Geometry: final body of the model. Coordinates: model frame, mm. A direction names the side the tool comes from. Coordinates: 2 decimals unless noted, no trailing zeros. Order: outer loops, then holes, each group sorted by start corner. A loop starts at its lowest first (then second) coordinate and runs counter-clockwise, first axis right, second up. Notation, with made-up numbers: M 71,23.5 L 85,23.5 A30 ccw 85,56.5 Z; hole C -2.75,-10.5 d7. An arc over 180 degrees is marked long. One line per question, with ' | ' between items.
from build123d import *

# Parameters (mm, degrees)
SKETCH1_R           = 3.7338
SKETCH1_R_2         = 2.6797
BOSS_EXTRUDE1_DEPTH = 1.1176
SHELL1_T            = -0.5715
BOSS_EXTRUDE2_DEPTH = 0.5588
SKETCH4_R           = 2.615046293
SKETCH4_R_2         = 2.107046293
BOSS_EXTRUDE3_DEPTH = 1.1176
BOSS_EXTRUDE4_DEPTH = 0.508
SKETCH7_W           = 0.381
SKETCH7_H           = 0.933727322


with BuildPart() as part:
    # Sketch1 → Boss-Extrude1 (new body)
    with BuildSketch(Plane(origin=(0, 0, 0), x_dir=(1, 0, 0), z_dir=(0, 1, 0))):
        with Locations(Location((0, 0, 0), (0, 0, 270))):
            Circle(SKETCH1_R)
        with Locations(Location((0, 0, 0), (0, 0, 270))):
            Circle(SKETCH1_R_2, mode=Mode.SUBTRACT)
    extrude(amount=-BOSS_EXTRUDE1_DEPTH)


with BuildPart() as body_2:
    # Sketch2 → Revolve1 (revolve)
    with BuildSketch(Plane.XY):
        with BuildLine():
            Line((0, -1.1176), (0, -20.9296))
            ThreePointArc((0, -20.9296), (-0.789505828, -20.640890822), (-1.206518449, -19.910977871))
            Line((-1.206518449, -19.910977871), (-2.770770199, -10.714786652))
            ThreePointArc((-2.770770199, -10.714786652), (-2.859495986, -10.068144543), (-2.906518408, -9.4171398))
            Line((-2.906518408, -9.4171398), (-3.2385, -1.1176))
            Line((-3.2385, -1.1176), (0, -1.1176))
        make_face()
    revolve(axis=Axis((0, -1.1176, 0), (0, -1, 0)))

    # Shell1
    shell1_openings = [body_2.faces().sort_by_distance(p)[0] for p in [
        (0, -1.1176, 0),
    ]]
    offset(amount=SHELL1_T, openings=shell1_openings, kind=Kind.INTERSECTION)


with BuildPart() as part_1:
    add(part.part)

    # Combine1: union body 2
    add(body_2.part)

    # Sketch3 → Boss-Extrude2 (add, symmetric)
    with BuildSketch(Plane.XY):
        with BuildLine():
            Line((3.7338, -1.1176), (4.365322861, -1.1176))
            Line((4.365322861, -1.1176), (5.180035681, -1.1176))
            ThreePointArc((5.180035681, -1.1176), (6.050241958, -0.247393722), (5.180035681, 0.622812555))
            Line((5.180035681, 0.622812555), (4.365322861, 0.622812555))
            Line((4.365322861, 0.622812555), (3.379294532, 0.622812555))
            Line((3.379294532, 0.622812555), (3.379294532, 0.112660745))
            Line((3.379294532, 0.112660745), (4.365322861, 0.112660745))
            Line((4.365322861, 0.112660745), (4.365322861, 0.36773665))
            Line((4.365322861, 0.36773665), (5.180035681, 0.36773665))
            ThreePointArc((5.180035681, 0.36773665), (5.795166053, -0.247393722), (5.180035681, -0.862524095))
            Line((5.180035681, -0.862524095), (4.365322861, -0.862524095))
            Line((4.365322861, -0.862524095), (4.365322861, -0.607448189))
            Line((4.365322861, -0.607448189), (3.379294532, -0.607448189))
            Line((3.379294532, -0.607448189), (3.379294532, -1.1176))
            Line((3.379294532, -1.1176), (3.7338, -1.1176))
        make_face()
    extrude(amount=BOSS_EXTRUDE2_DEPTH, both=True)



with BuildPart() as body_2_2:
    # Sketch4 → Boss-Extrude3 (new body)
    with BuildSketch(Plane.XZ.offset(-0.112660745)):
        with Locations(Location((0, 0, 0), (0, 0, 270))):
            Circle(SKETCH4_R)
        with Locations(Location((0, 0, 0), (0, 0, 270))):
            Circle(SKETCH4_R_2, mode=Mode.SUBTRACT)
    extrude(amount=BOSS_EXTRUDE3_DEPTH)

    # Sketch5 → Revolve2 (revolve)
    with BuildSketch(Plane.XY):
        with BuildLine():
            Line((-2.615046293, 0.112660745), (-2.615046293, 1.160799378))
            ThreePointArc((-2.615046293, 1.160799378), (-1.849116967, 3.009916345), (0, 3.775845671))
            Line((0, 3.775845671), (0, 3.267845671))
            ThreePointArc((0, 3.267845671), (-1.489906722, 2.6507061), (-2.107046293, 1.160799378))
            Line((-2.107046293, 1.160799378), (-2.107046293, 0.112660745))
            Line((-2.107046293, 0.112660745), (-2.107046293, 0.047504608))
            Line((-2.107046293, 0.047504608), (-2.615046293, 0.047504608))
            Line((-2.615046293, 0.047504608), (-2.615046293, 0.112660745))
        make_face()
    revolve(axis=Axis((0, 3.775845671, 0), (0, -1, 0)))


with BuildPart() as part_2:
    add(part_1.part)

    add(body_2_2.part)  # Boss-Extrude4 merges body 2 2
    # Sketch6 → Boss-Extrude4 (add)
    with BuildSketch(Plane.XZ.offset(-0.112660745)):
        with BuildLine():
            Line((-2.179935272, -3.062591525), (-4.50743423, -1.405890971))
            ThreePointArc((-4.50743423, -1.405890971), (-5.2324, 0), (-4.50743423, 1.405890971))
            Line((-4.50743423, 1.405890971), (-2.179935272, 3.062591525))
            ThreePointArc((-2.179935272, 3.062591525), (3.7592, 0), (-2.179935272, -3.062591525))
        make_face()
    extrude(amount=-BOSS_EXTRUDE4_DEPTH)

    # Sketch7 → Revolve3 (revolve)
    with BuildSketch(Plane.XY, mode=Mode.PRIVATE) as revolve3_sk:
        with Locations((-0.1905, -21.097736339)):
            Rectangle(SKETCH7_W, SKETCH7_H)
    revolve(revolve3_sk.sketch.rotate(Axis((0, -20.630872678, 0), (0, -1, 0)), 270), axis=Axis((0, -20.630872678, 0), (0, -1, 0)))


solid = part_2.part
1. Section D-D, the plane y = 2.75. Output: boundary loops of the cut face in (x, z), and give its area (3 significant figures).
Response values:
outline: C 0,0 d4.15; hole C 0,0 d2.77 | area: 7.54 mm^2
2. Section C-C, the plane y = -14.75. Output: boundary loops of the cut face in (x, z).
Response values:
outline: C 0,0 d4.17; hole C 0,0 d3.01
3. Access query for faces 4 (the face through (2.075, 0.895, 1.591)), 5 (the face through (2.44, -5.21, 1.87)), 6 (the face through (5.795, -0.234, 0.008)), 7 (the face through (0, 0.621, 0)). Directions: +Z, -Z, +X, -X, +Y, -Y. A direction counts if a zero-diameter tool reaches every point of the face in a straight line with its end or side. Return the directions, or none.
Response values:
face 4: +Y | face 5: -Y | face 6: +Z, -Z | face 7: none
4. Material intervals for line 1 (X direction, y = 0.95, z = 0); line 2 (X direction, y = -16, z = 0), sorted ascending. Write a range as [from, to].
Response values:
line 1: x = [-2.62, -2.11], [2.11, 2.62] | line 2: x = [-1.87, -1.29], [1.29, 1.87]
5. Draft query along X for faces 1 (the face through (5, 0.368, 0)), 2 (the face through (1.52, 0.36, -3.44)), 3 (the face through (4, 0.623, 0)). Return one class per face: pulls with the +X half, pulls with the -X half, needs draft (parallel to the pull), parting line crosses it, or undercut.
Response values:
face 1: undercut | face 2: parting line crosses it | face 3: needs draft
6. Pin query (flat end, axial travel): P1, Ø1.2, axis at x = 4.5, z = 0, coming from the +Y side; P2, Ø2, axis at x = -2.5, z = -2, coming from the +Y side; P3, Ø1.5, axis at x = 5, z = -2, coming from the -Y side; P4, Ø1.9, axis at x = 4, y = 0, coming from the -Z side. Return the tip coordinate at first contact, or that it passes through.
Response values:
P1: stops at y = 0.62 | P2: stops at y = 2.57 | P3: passes through | P4: stops at z = -2.19
7. Section A-A, the plane x = 0. Give the number of separate pieces and of enclosed holes in the cut face, and give its area (3 significant figures).
Response values:
separate pieces: 2 | enclosed holes: 1 | area: 35.2 mm^2
